Could you check a few things on this drawing? It's one solid part, dimensions in mm from its lowest x, y, z. Round coordinates to 2 decimals unless told otherwise and drop trailing zeros. Write each loop counter-clockwise with the first axis right and the second up, starting at its lowest first coordinate (ties: lowest second). Pieces come first, ordered by that corner, then holes. Notation, with made-up numbers: (-3, 66.25) -> (22, 66.25) arc R8 cw to (22, 73.25) -> close; hole circle Ø4 at (-9.75, 62.5). An arc over 180 degrees is marked (long way). Answer in a Markdown table with one row per item.
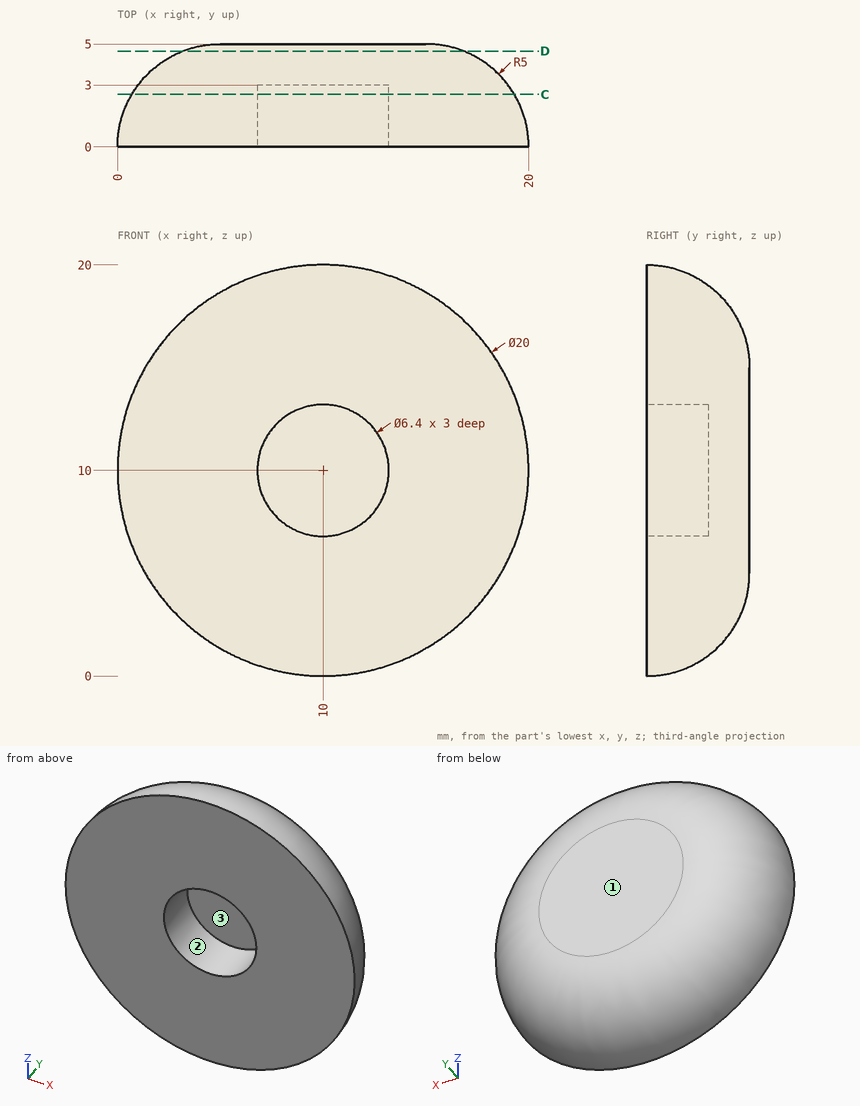
1) Imagine slicing it at C-C, the plane y = 2.55. Please give me the cut outline in (x, z).
Findings:
| item | result |
|---|---|
| outline | circle Ø18.6 at (10, 10); hole circle Ø6.4 at (10, 10) |
2) Thinking about a two-plate mould opening in X: for the marked faces 1, 2 and 3, which applies, +X half, -X half, draft (parallel to the pull), parting line (faces both ways), or undercut?
Findings:
| item | result |
|---|---|
| face 1 | draft |
| face 2 | undercut |
| face 3 | undercut |
3) For pin 1 (10 mm diameter, centred on x = 6, z = 3.5, fed in from +Y); pin 2 (1 mm diameter, centred on x = 9, y = 2, fed in from -Z); pin 3 (1 mm diameter, centred on x = 3.5, z = 12, fed in from +Y), each with a flat end and sliding along its axis, tell me the tip position at first contact or that it passes through.
Findings:
| item | result |
|---|---|
| pin 1 | stops at y = 5 |
| pin 2 | stops at z = 0.27 |
| pin 3 | stops at y = 4.83 |
4) Imagine slicing it at D-D, the plane y = 4.65. Please give me the cut outline in (x, z), plus the area to 3 significant figures.
Findings:
| item | result |
|---|---|
| outline | circle Ø13.68 at (10, 10) |
| area | 147 mm^2 |
5) Please list where these lines run through material, in increasing order: line 1 (Z direction, x = 10, y = 2.1); line 2 (Z direction, x = 10, y = 0.8); line 3 (Z direction, x = 18.5, y = 0.75).
Findings:
| item | result |
|---|---|
| line 1 | z = 0.46 to 6.8, 13.2 to 19.54 |
| line 2 | z = 0.06 to 6.8, 13.2 to 19.94 |
| line 3 | z = 4.84 to 15.16 |
